Source: CAD feature listing. Evaluate the final solid. Frame: model axes, mm. Face numbers are marked on the shaded views. A direction names the side the tool comes from. Round coordinates to 2 decimals unless told otherwise and drop trailing zeros. Loops run counter-clockwise (first coordinate to the right, second up) from the corner with the lowest first, then second, coordinate; pieces in that order, holes last. Notation, with made-up numbers: M -39.75,9.25 L -1.75,9.25 A22 ccw -1.75,30.25 Z; hole C 75.25,25 d6. An arc over 180 degrees is marked long. Answer as CSV lines item,"result". Start each with the question number.
```python
from build123d import *

# Parameters (mm, degrees)
BOSS_EXTRUDE8_DEPTH  = 4
BOSS_EXTRUDE10_DEPTH = 8
BOSS_EXTRUDE11_DEPTH = 4
SKETCH14_R           = 2.7
SKETCH14_W           = 20.4
SKETCH14_H           = 20.4
CUT_EXTRUDE1_DEPTH   = 12


with BuildPart() as part:
    # Sketch11 → Boss-Extrude8 (new body)
    with BuildSketch(Plane(origin=(0, 0, 0), x_dir=(1, 0, 0), z_dir=(0, 1, 0))):
        with BuildLine():
            Line((27.930717857, -16.617009358), (41.012193309, -29.69848481))
            Line((41.012193309, -29.69848481), (43.08274567, -37.42589142))
            Line((43.08274567, -37.42589142), (37.42589142, -43.08274567))
            Line((37.42589142, -43.08274567), (29.69848481, -41.012193309))
            Line((29.69848481, -41.012193309), (16.617009358, -27.930717857))
            ThreePointArc((16.617009358, -27.930717857), (0, -32.5), (-16.617009358, -27.930717857))
            Line((-16.617009358, -27.930717857), (-29.69848481, -41.012193309))
            Line((-29.69848481, -41.012193309), (-37.42589142, -43.08274567))
            Line((-37.42589142, -43.08274567), (-43.08274567, -37.42589142))
            Line((-43.08274567, -37.42589142), (-41.012193309, -29.69848481))
            Line((-41.012193309, -29.69848481), (-27.930717857, -16.617009358))
            ThreePointArc((-27.930717857, -16.617009358), (-32.5, 0), (-27.930717857, 16.617009358))
            Line((-27.930717857, 16.617009358), (-41.012193309, 29.69848481))
            Line((-41.012193309, 29.69848481), (-43.08274567, 37.42589142))
            Line((-43.08274567, 37.42589142), (-37.42589142, 43.08274567))
            Line((-37.42589142, 43.08274567), (-29.69848481, 41.012193309))
            Line((-29.69848481, 41.012193309), (-16.617009358, 27.930717857))
            ThreePointArc((-16.617009358, 27.930717857), (0, 32.5), (16.617009358, 27.930717857))
            Line((16.617009358, 27.930717857), (29.69848481, 41.012193309))
            Line((29.69848481, 41.012193309), (37.42589142, 43.08274567))
            Line((37.42589142, 43.08274567), (43.08274567, 37.42589142))
            Line((43.08274567, 37.42589142), (41.012193309, 29.69848481))
            Line((41.012193309, 29.69848481), (27.930717857, 16.617009358))
            ThreePointArc((27.930717857, 16.617009358), (32.5, 0), (27.930717857, -16.617009358))
        make_face()
    extrude(amount=BOSS_EXTRUDE8_DEPTH)

    # Sketch12 → Boss-Extrude10 (add)
    with BuildSketch(Plane(origin=(0, 4, 0), x_dir=(1, 0, 0), z_dir=(0, 1, 0))):
        with BuildLine():
            Line((38.890872967, 31.819805152), (41.012193309, 29.69848481))
            Line((41.012193309, 29.69848481), (26.10190255, 14.788194051))
            ThreePointArc((26.10190255, 14.788194051), (27.250407583, 12.546524879), (28.206823147, 10.216414633))
            Line((28.206823147, 10.216414633), (30.585684682, 10.9893536))
            ThreePointArc((30.585684682, 10.9893536), (30.90933678, 10.043052317), (31.203718671, 9.087240568))
            Line((31.203718671, 9.087240568), (28.824857136, 8.3143016))
            ThreePointArc((28.824857136, 8.3143016), (29.630650218, 4.693033951), (29.983328701, 1))
            Line((29.983328701, 1), (32.484611742, 1))
            ThreePointArc((32.484611742, 1), (32.5, 0), (32.484611742, -1))
            Line((32.484611742, -1), (29.983328701, -1))
            ThreePointArc((29.983328701, -1), (29.630650218, -4.693033951), (28.824857136, -8.3143016))
            Line((28.824857136, -8.3143016), (31.203718671, -9.087240568))
            ThreePointArc((31.203718671, -9.087240568), (30.90933678, -10.043052317), (30.585684682, -10.9893536))
            Line((30.585684682, -10.9893536), (28.206823147, -10.216414633))
            ThreePointArc((28.206823147, -10.216414633), (27.250407583, -12.546524879), (26.10190255, -14.788194051))
            Line((26.10190255, -14.788194051), (41.012193309, -29.69848481))
            Line((41.012193309, -29.69848481), (38.890872965, -31.819805153))
            ThreePointArc((38.890872965, -31.819805153), (38.890872965, -38.890872967), (31.819805152, -38.890872967))
            Line((31.819805152, -38.890872967), (29.69848481, -41.012193309))
            Line((29.69848481, -41.012193309), (14.788194051, -26.10190255))
            ThreePointArc((14.788194051, -26.10190255), (12.546524879, -27.250407583), (10.216414633, -28.206823147))
            Line((10.216414633, -28.206823147), (10.9893536, -30.585684682))
            ThreePointArc((10.9893536, -30.585684682), (10.043052317, -30.90933678), (9.087240568, -31.203718671))
            Line((9.087240568, -31.203718671), (8.3143016, -28.824857136))
            ThreePointArc((8.3143016, -28.824857136), (4.693033951, -29.630650218), (1, -29.983328701))
            Line((1, -29.983328701), (1, -32.484611742))
            ThreePointArc((1, -32.484611742), (0, -32.5), (-1, -32.484611742))
            Line((-1, -32.484611742), (-1, -29.983328701))
            ThreePointArc((-1, -29.983328701), (-4.693033951, -29.630650218), (-8.3143016, -28.824857136))
            Line((-8.3143016, -28.824857136), (-9.087240568, -31.203718671))
            ThreePointArc((-9.087240568, -31.203718671), (-10.043052317, -30.90933678), (-10.9893536, -30.585684682))
            Line((-10.9893536, -30.585684682), (-10.216414633, -28.206823147))
            ThreePointArc((-10.216414633, -28.206823147), (-12.546524879, -27.250407583), (-14.788194051, -26.10190255))
            Line((-14.788194051, -26.10190255), (-29.69848481, -41.012193309))
            Line((-29.69848481, -41.012193309), (-31.819805153, -38.890872965))
            ThreePointArc((-31.819805153, -38.890872965), (-38.890872967, -38.890872965), (-38.890872967, -31.819805152))
            Line((-38.890872967, -31.819805152), (-41.012193309, -29.69848481))
            Line((-41.012193309, -29.69848481), (-26.10190255, -14.788194051))
            ThreePointArc((-26.10190255, -14.788194051), (-27.250407583, -12.546524879), (-28.206823147, -10.216414633))
            Line((-28.206823147, -10.216414633), (-30.585684682, -10.9893536))
            ThreePointArc((-30.585684682, -10.9893536), (-30.90933678, -10.043052317), (-31.203718671, -9.087240568))
            Line((-31.203718671, -9.087240568), (-28.824857136, -8.3143016))
            ThreePointArc((-28.824857136, -8.3143016), (-29.630650218, -4.693033951), (-29.983328701, -1))
            Line((-29.983328701, -1), (-32.484611742, -1))
            ThreePointArc((-32.484611742, -1), (-32.5, 0), (-32.484611742, 1))
            Line((-32.484611742, 1), (-29.983328701, 1))
            ThreePointArc((-29.983328701, 1), (-29.630650218, 4.693033951), (-28.824857136, 8.3143016))
            Line((-28.824857136, 8.3143016), (-31.203718671, 9.087240568))
            ThreePointArc((-31.203718671, 9.087240568), (-30.90933678, 10.043052317), (-30.585684682, 10.9893536))
            Line((-30.585684682, 10.9893536), (-28.206823147, 10.216414633))
            ThreePointArc((-28.206823147, 10.216414633), (-27.250407583, 12.546524879), (-26.10190255, 14.788194051))
            Line((-26.10190255, 14.788194051), (-41.012193309, 29.69848481))
            Line((-41.012193309, 29.69848481), (-38.890872965, 31.819805153))
            ThreePointArc((-38.890872965, 31.819805153), (-38.890872965, 38.890872967), (-31.819805152, 38.890872967))
            Line((-31.819805152, 38.890872967), (-29.69848481, 41.012193309))
            Line((-29.69848481, 41.012193309), (-14.788194051, 26.10190255))
            ThreePointArc((-14.788194051, 26.10190255), (-12.546524879, 27.250407583), (-10.216414633, 28.206823147))
            Line((-10.216414633, 28.206823147), (-10.9893536, 30.585684682))
            ThreePointArc((-10.9893536, 30.585684682), (-10.043052317, 30.90933678), (-9.087240568, 31.203718671))
            Line((-9.087240568, 31.203718671), (-8.3143016, 28.824857136))
            ThreePointArc((-8.3143016, 28.824857136), (-4.693033951, 29.630650218), (-1, 29.983328701))
            Line((-1, 29.983328701), (-1, 32.484611742))
            ThreePointArc((-1, 32.484611742), (0, 32.5), (1, 32.484611742))
            Line((1, 32.484611742), (1, 29.983328701))
            ThreePointArc((1, 29.983328701), (4.693033951, 29.630650218), (8.3143016, 28.824857136))
            Line((8.3143016, 28.824857136), (9.087240568, 31.203718671))
            ThreePointArc((9.087240568, 31.203718671), (10.043052317, 30.90933678), (10.9893536, 30.585684682))
            Line((10.9893536, 30.585684682), (10.216414633, 28.206823147))
            ThreePointArc((10.216414633, 28.206823147), (12.546524879, 27.250407583), (14.788194051, 26.10190255))
            Line((14.788194051, 26.10190255), (29.69848481, 41.012193309))
            Line((29.69848481, 41.012193309), (31.819805153, 38.890872965))
            ThreePointArc((31.819805153, 38.890872965), (38.890872967, 38.890872965), (38.890872967, 31.819805152))
        make_face()
    extrude(amount=BOSS_EXTRUDE10_DEPTH)

    # Sketch13 → Boss-Extrude11 (add)
    with BuildSketch(Plane(origin=(0, 12, 0), x_dir=(1, 0, 0), z_dir=(0, 1, 0))):
        with BuildLine():
            Line((27.930717857, -16.617009358), (41.012193309, -29.69848481))
            Line((41.012193309, -29.69848481), (43.08274567, -37.42589142))
            Line((43.08274567, -37.42589142), (37.42589142, -43.08274567))
            Line((37.42589142, -43.08274567), (29.69848481, -41.012193309))
            Line((29.69848481, -41.012193309), (16.617009358, -27.930717857))
            ThreePointArc((16.617009358, -27.930717857), (0, -32.5), (-16.617009358, -27.930717857))
            Line((-16.617009358, -27.930717857), (-29.69848481, -41.012193309))
            Line((-29.69848481, -41.012193309), (-37.42589142, -43.08274567))
            Line((-37.42589142, -43.08274567), (-43.08274567, -37.42589142))
            Line((-43.08274567, -37.42589142), (-41.012193309, -29.69848481))
            Line((-41.012193309, -29.69848481), (-27.930717857, -16.617009358))
            ThreePointArc((-27.930717857, -16.617009358), (-32.5, 0), (-27.930717857, 16.617009358))
            Line((-27.930717857, 16.617009358), (-41.012193309, 29.69848481))
            Line((-41.012193309, 29.69848481), (-43.08274567, 37.42589142))
            Line((-43.08274567, 37.42589142), (-37.42589142, 43.08274567))
            Line((-37.42589142, 43.08274567), (-29.69848481, 41.012193309))
            Line((-29.69848481, 41.012193309), (-16.617009358, 27.930717857))
            ThreePointArc((-16.617009358, 27.930717857), (0, 32.5), (16.617009358, 27.930717857))
            Line((16.617009358, 27.930717857), (29.69848481, 41.012193309))
            Line((29.69848481, 41.012193309), (37.42589142, 43.08274567))
            Line((37.42589142, 43.08274567), (43.08274567, 37.42589142))
            Line((43.08274567, 37.42589142), (41.012193309, 29.69848481))
            Line((41.012193309, 29.69848481), (27.930717857, 16.617009358))
            ThreePointArc((27.930717857, 16.617009358), (32.5, 0), (27.930717857, -16.617009358))
        make_face()
    extrude(amount=BOSS_EXTRUDE11_DEPTH)

    # Sketch14 → Cut-Extrude1 (cut)
    with BuildSketch(Plane(origin=(0, 16, 0), x_dir=(1, 0, 0), z_dir=(0, 1, 0))):
        with Locations(Location((-35.355339059, 35.355339059, 0), (0, 0, 270))):
            Circle(SKETCH14_R)
        with Locations(Location((35.355339059, 35.355339059, 0), (0, 0, 270))):
            Circle(SKETCH14_R)
        with Locations(Location((35.355339059, -35.355339059, 0), (0, 0, 270))):
            Circle(SKETCH14_R)
        with Locations(Location((-35.355339059, -35.355339059, 0), (0, 0, 270))):
            Circle(SKETCH14_R)
        Rectangle(SKETCH14_W, SKETCH14_H)
    extrude(amount=-CUT_EXTRUDE1_DEPTH, mode=Mode.SUBTRACT)


solid = part.part
```
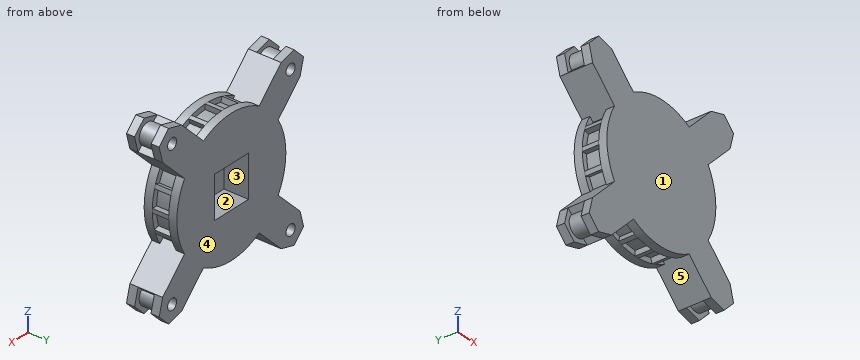
1) Contact query for flat-ended pins moving along their axis: pin 1 Ø6 at (x, y) = (-3.5, 11.5) entering from +Z; pin 2 Ø3 at (x, y) = (-5, 2.5) entering from -Z; pin 3 Ø2 at (x, z) = (34, -21) entering from +Y; pin 4 Ø2 at (y, z) = (10, -31) entering from +X. Output: stop coordinate, or through.
2) Section B-B, the plane x = 34. Return loops of the section in (y, z).
3) Section C-C, the plane x = 4. Return loops of the section in (y, z), and give its area (3 significant figures).
4) Section A-A, the plane y = 2.75. Return loops of the section in (x, z).
5) Ray query, line 1 along Y through (x, z) = (6, -29.5); line 2 along X through (y, z) = (13.5, -35.5); line 3 along Z through (x, y) = (-39, 6). Return the intervals inside material, ascending.
6) Access query for the marked faces 1 and 2. Directions: +Z, -Z, +X, -X, +Y, -Y. A direction counts if a zero-diameter tool reaches every point of the face in a straight line with its end or side. Return the directions, or none.
7) Section D-D, the plane y = 7.5. Give the number of separate pieces and of enclosed holes in the cut face, and give its area (3 significant figures).
8) Mould query, pull axis Z, two halves, no side actions, for the marked faces 3, 4 and 5. Classes: pulls with the +Z half, pulls with the -Z half, needs draft (parallel to the pull), parting line crosses it, or undercut.
Findings below:
1,pin 1,"z = 32.5"
1,pin 2,"z = -32.31"
1,pin 3,"through"
1,pin 4,"x = 40.71"
2,outline,"M 0,-42.16 L 4,-42.16 L 4,-40.17 L 12,-40.17 L 12,-42.16 L 16,-42.16 L 16,-37.69 L 4,-37.69 L 4,-33.02 L 16,-33.02 L 16,-22.69 L 0,-22.69 Z; M 0,22.69 L 16,22.69 L 16,33.02 L 4,33.02 L 4,37.69 L 16,37.69 L 16,42.16 L 12,42.16 L 12,40.17 L 4,40.17 L 4,42.16 L 0,42.16 Z"
3,outline,"M 0,-32.25 L 4,-32.25 L 4,-29.73 L 12,-29.73 L 12,-32.25 L 16,-32.25 L 16,-10.2 L 4,-10.2 L 4,10.2 L 16,10.2 L 16,32.25 L 12,32.25 L 12,29.73 L 4,29.73 L 4,32.25 L 0,32.25 Z"
3,area,"747 mm²"
4,outline,"M -43.08,-37.43 L -37.43,-43.08 L -29.7,-41.01 L -16.62,-27.93 A32.5 ccw 16.62,-27.93 L 29.7,-41.01 L 37.43,-43.08 L 43.08,-37.43 L 41.01,-29.7 L 27.93,-16.62 A32.5 ccw 27.93,16.62 L 41.01,29.7 L 43.08,37.43 L 37.43,43.08 L 29.7,41.01 L 16.62,27.93 A32.5 ccw -16.62,27.93 L -29.7,41.01 L -37.43,43.08 L -43.08,37.43 L -41.01,29.7 L -27.93,16.62 A32.5 ccw -27.93,-16.62 L -41.01,-29.7 Z"
5,line 1,"0 to 4, 12 to 16"
5,line 2,"-42.57 to -38.05, -32.66 to -24.19, 24.19 to 32.66, 38.05 to 42.57"
5,line 3,"-38.78 to -31.93, -31.71 to -27.69, 27.69 to 31.71, 31.93 to 38.78"
6,face 1,"+Z, -Z, +X, -X, -Y"
6,face 2,"+Y"
7,separate pieces,"1"
7,enclosed holes,"5"
7,area,"3,840 mm²"
8,face 3,"undercut"
8,face 4,"needs draft"
8,face 5,"pulls with the -Z half"
